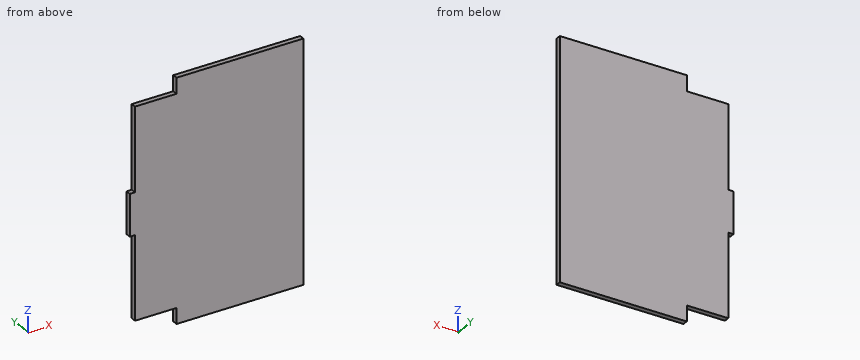
```python
from build123d import *

# Parameters (mm, degrees)
BOSS_EXTRUDE1_DEPTH = 3.175
SKETCH2_W           = 29.21
SKETCH2_H           = 146.05
CUT_EXTRUDE1_DEPTH  = 101.731234192


with BuildPart() as part:
    # Sketch1 → Boss-Extrude1 (new body)
    with BuildSketch(Plane(origin=(0, 0, 0), x_dir=(1, 0, 0), z_dir=(0, 1, 0))):
        Polygon((-40.736256602, -73.025), (59.786256602, -73.025), (59.786256602, -63.5), (66.136256602, -63.5), (66.136256602, 63.5), (59.786256602, 63.5), (59.786256602, 73.025), (-40.736256602, 73.025), (-40.736256602, 63.5), (-66.136256602, 63.5), (-66.136256602, 12.7), (-69.311256602, 12.7), (-69.311256602, -12.7), (-66.136256602, -12.7), (-66.136256602, -63.5), (-40.736256602, -63.5), align=None)
    extrude(amount=BOSS_EXTRUDE1_DEPTH)

    # Sketch2 → Cut-Extrude1 (cut, through all)
    with BuildSketch(Plane.XZ):
        with Locations((51.531256602, 0)):
            Rectangle(SKETCH2_W, SKETCH2_H)
    extrude(amount=-CUT_EXTRUDE1_DEPTH, mode=Mode.SUBTRACT)


solid = part.part
```
Here's how the part is built. I have some questions about the finished solid (model axes, mm). Coordinates: 2 decimals unless noted, no trailing zeros. Order: outer loops, then holes, each group sorted by start corner. A loop starts at its lowest first (then second) coordinate and runs counter-clockwise, first axis right, second up.
1) Will these pins go through, and if not, where does the flat tip stop? pin 1 (1 mm diameter, centred on x = -67.5, y = 1.5, fed in from +Z); pin 2 (1.6 mm diameter, centred on y = 2, z = 69.5, fed in from -X); pin 3 (1.6 mm diameter, centred on y = 1.5, z = -42.5, fed in from -X).
2) Imagine slicing it at A-A on y = 1.9. List the corners of the cut face in (x, z) for me (3 decimals), and give its area (3 significant figures).
3) Imagine slicing it at B-B on x = -53.5. List the corners of the cut face in (y, z) for me (3 decimals), and give its area (3 significant figures).
4) I need wall thicknesses on line 1 (X direction, y = 1.65, z = 15); line 2 (Z direction, x = -47, y = 2.6); line 3 (X direction, y = 0.6, z = 67). Which ranges of each line are inside material? Lowest first, please.
5) Imagine slicing it at C-C on z = -22.5. List the corners of the cut face in (x, y) for me (3 decimals), and give its area (3 significant figures).
Response values:
1. pin 1: stops at z = 12.7
1. pin 2: stops at x = -40.74
1. pin 3: stops at x = -66.14
2. outline: (-69.311, -12.7) - (-66.136, -12.7) - (-66.136, -63.5) - (-40.736, -63.5) - (-40.736, -73.025) - (36.926, -73.025) - (36.926, 73.025) - (-40.736, 73.025) - (-40.736, 63.5) - (-66.136, 63.5) - (-66.136, 12.7) - (-69.311, 12.7) - close
2. area: 14,600 mm2
3. outline: (0, -63.5) - (3.175, -63.5) - (3.175, 63.5) - (0, 63.5) - close
3. area: 403 mm2
4. line 1: x = -66.14 to 36.93
4. line 2: z = -63.5 to 63.5
4. line 3: x = -40.74 to 36.93
5. outline: (-66.136, 0) - (36.926, 0) - (36.926, 3.175) - (-66.136, 3.175) - close
5. area: 327 mm2
